Can you work these out from the model? Positions are in its coordinate system, mm. Face numbers are marked on the shaded views. Round coordinates to 2 decimals unless told otherwise and drop trailing zeros. Order: outer loops, then holes, each group sorted by start corner. A loop starts at its lowest first (then second) coordinate and runs counter-clockwise, first axis right, second up. Notation, with made-up numbers: (75, -37) - (128, -37) arc R7 ccw to (128, -28) - close; hole circle Ø10 at (52, -39.75). An arc over 180 degrees is marked (long way). Write item = value, one per line.
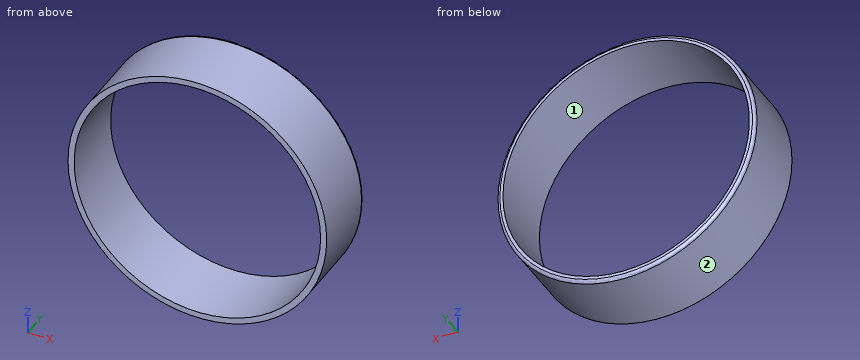
Autodesk Fusion 360 part; units mm, degrees
sketch "Sketch3" plane through (0, 0, 0) normal (0, 1, 0) x (1, 0, 0)
  circle A0 centre (0, 0) radius 40.3
  circle A1 centre (0, 0) radius 42.3
  line L0 (30, -20) -> (-30, -20)
  line L1 (-30, -20) -> (-30, 20)
  line L2 (-30, 20) -> (30, 20)
  line L3 (30, 20) -> (30, -20)
  line L4 (30, -20) -> (-30, 20) construction
  line L5 (-30, -20) -> (30, 20) construction
  dimension "d13" = 80.6
  dimension "d14" = 2
  dimension "d34" = 60
  dimension "d35" = 40
extrude "Extrude3" add sketch "Sketch3" along normal blind 21 contours A1
sketch "Sketch4" plane through (0, 0, 0) normal (0, 0, 1) x (1, 0, 0)
  line L0 (-49.5, 21) -> (-47.3, 21)
  line L1 (49.5, 21) -> (47.3, 21)
  line L2 (-47.3, 21) -> (-47.3, 25.1334)
  line L3 (47.3, 21) -> (47.3, 25.1334)
  line L4 (47.3, 27) -> (47.3, 25)
  arc A0 (47.3, 25) -> (-47.3, 25) centre (0, -131.3064) ccw
  line L5 (47.3, 21) -> (45.3, 21)
  line L6 (45.3, 21) -> (45.3, 25.5913)
  line L7 (-47.3, 21) -> (-45.3, 21)
  line L8 (-45.3, 21) -> (-45.3, 25.5913)
  arc A1 (0, 32) -> (-47.3, 25) centre (0, -131.3064) ccw
  line L9 (0, 32) -> (0, 34)
  arc A2 (45.4965, 27.5344) -> (-45.4965, 27.5344) centre (0, -129.3064) ccw
  arc A3 (-45.4965, 27.5344) -> (-47.3, 25.1334) centre (-44.8, 25.1334) ccw
  arc A4 (47.3, 25.1334) -> (45.4965, 27.5344) centre (44.8, 25.1334) ccw
  line L10 (0, 21) -> (-2.5, 21)
  line L11 (-2.5, 21) -> (-2.5, 31.9809)
  line L12 (0, 21) -> (0, 32)
  line L13 (-42, 21) -> (-39.8, 21)
  line L14 (42, 21) -> (39.8, 21)
  line L15 (39.8, 21) -> (39.8, 27.0759)
  line L16 (-39.8, 21) -> (-39.8, 27.0759)
  line L17 (-39.8, 21) -> (-37.8, 21)
  line L18 (-37.8, 21) -> (-37.8, 27.5651)
  line L19 (37.8, 21) -> (37.8, 27.5651)
  line L20 (37.8, 21) -> (39.8, 21)
  line L21 (-39.8, 27.0759) -> (-39.8, 29.0759)
  line L22 (39.8, 27.0759) -> (39.8, 29.0759)
  line L23 (-39.8, 27.0759) -> (0, 27.0759)
  line L24 (0, 27.0759) -> (0, 34)
  point P0 (-47.3, 27)
  dimension "d17" = 2.2
  dimension "d18" = 2.2
  dimension "d19" = 6
  dimension "d20" = 6
  dimension "d22" = 2
  dimension "d23" = 2
  dimension "d24" = 2
  dimension "d25" = 2
  dimension "d26" = 2
  dimension "d27" = 2.5
  dimension "d28" = 2.5
  dimension "d36" = 2.2
  dimension "d37" = 2.2
  dimension "d38" = 2
  dimension "d39" = 2
sketch "Sketch5" plane through (0, 0, 0) normal (0, -1, 0) x (1, 0, 0)
  circle A0 centre (0, 0) radius 40.3
  circle A1 centre (0, 0) radius 42.3
extrude "Extrude4" add sketch "Sketch5" along normal blind 2 contours A0 | A1
fillet "Fillet2" radius 1 1 edges at (-39.4374, 21, 15.2963)
sketch "Sketch6" plane through (0, -2, 0) normal (0, -1, 0) x (1, 0, 0)
  line L0 (20, 27.5) -> (-20, 27.5)
  line L1 (-20, 27.5) -> (-20, -27.5)
  line L2 (-20, -27.5) -> (20, -27.5)
  line L3 (20, -27.5) -> (20, 27.5)
  line L4 (20, 27.5) -> (-20, -27.5) construction
  line L5 (-20, 27.5) -> (20, -27.5) construction
  circle A0 centre (0, 0) radius 42.3
  dimension "d41" = 55
  dimension "d42" = 40
sketch "Sketch7" plane through (0, -2, 0) normal (0, -1, 0) x (1, 0, 0)
  circle A0 centre (0, 0) radius 42.3
sketch "Sketch8" plane through (0, -2, 0) normal (0, -1, 0) x (1, 0, 0)
  circle A0 centre (0, 0) radius 42.3
sketch "Sketch9" plane through (0, 0, 0) normal (0, 0, 1) x (1, 0, 0)
sketch "Sketch10" plane through (0, -2, 0) normal (0, -1, 0) x (1, 0, 0)
  circle A0 centre (0, 0) radius 42.3
  circle A1 centre (0, 0) radius 40.3
  dimension "d43" = -2
extrude "Extrude5" cut sketch "Sketch10" against normal blind 3 contours A1
sketch "Sketch11" plane through (0, 21, 0) normal (0, 1, 0) x (-1, 0, 0)
  circle A0 centre (0, 0) radius 40.3
  circle A1 centre (0, 0) radius 41.3
  line L0 (42, 0) -> (40.3, 0)
  line L1 (40.3, 0) -> (39.3, 0)
  circle A2 centre (0, 0) radius 39.3
  dimension "d46" = 1
extrude "Extrude6" [suppressed]
fillet "Fillet3" [suppressed]
equation "d17 = 2 mm + 0.2 mm"
equation "d18 = 2 mm + 0.2 mm"
equation "d36 = 2 mm + 0.2 mm"
equation "d37 = 2 mm + 0.2 mm"
(1) Will these pins go through, and if not, where does the flat tip stop? P1, Ø3, axis at y = 9, z = -23.5, coming from the -X side; P2, Ø5, axis at x = -10.5, y = 3, coming from the -Z side; P3, Ø8, axis at x = -12.5, y = 12, coming from the -Z side.
Computed:
P1 = -36.13
P2 = -41.54
P3 = -41.44
(2) If we section it at B-B (z = 0): Write out the boundary of the cut face in (x, y).
Computed:
outline = (-42.3, -2) - (-40.3, -2) - (-40.3, 21) - (-41.3, 21) arc R1 ccw to (-42.3, 20) - close; (40.3, -2) - (42.3, -2) - (42.3, 20) arc R1 ccw to (41.3, 21) - (40.3, 21) - close
(3) If we section it at C-C (y = 2.5): Write out the boundary of the cut face in (x, z).
Computed:
outline = circle Ø84.6 at (0, 0); hole circle Ø80.6 at (0, 0)
(4) Thinking about a two-plate mould opening in X: for the marked faces 1 and 2, which applies, +X half, -X half, draft (parallel to the pull), parting line (faces both ways), or undercut?
Computed:
face_1 = undercut
face_2 = parting line
(5) If we section it at A-A (x = 0): Write out the boundary of the cut face in (y, z), plus the area to 3 significant figures.
Computed:
outline = (-2, -42.3) - (20, -42.3) arc R1 ccw to (21, -41.3) - (21, -40.3) - (-2, -40.3) - close; (-2, 40.3) - (21, 40.3) - (21, 41.3) arc R1 ccw to (20, 42.3) - (-2, 42.3) - close
area = 91.6 mm^2
(6) If I drill on line 1 (Z direction, x = 0, y = 15.75); line 2 (X direction, y = 0.5, z = 8), over which ranges is the centre line in solid material (lowest first)? Write a range as from..to.
Computed:
line_1 = -42.3..-40.3, 40.3..42.3
line_2 = -41.54..-39.5, 39.5..41.54
